Design review of the part built by this model. Coordinates are the model's own, in mm. A direction names the side the tool comes from. Round coordinates to 2 decimals unless told otherwise and drop trailing zeros. Loops run counter-clockwise (first coordinate to the right, second up) from the corner with the lowest first, then second, coordinate; pieces in that order, holes last. Notation, with made-up numbers: M 66,-31.75 L 93,-31.75 A25 ccw 93,-4.75 Z; hole C 16.5,-3 d9. An arc over 180 degrees is marked long. Answer as CSV lines item,"result". Start each with the question number.
Autodesk Fusion 360 part; units mm, degrees
sketch "Sketch1" plane through (0, 0, 0) normal (0, 0, 1) x (1, 0, 0)
  line L0 (5.4842, 0) -> (306.4842, 0)
  line L1 (311.4842, 5) -> (311.4842, 200)
  line L2 (306.4842, 205) -> (5.4842, 205)
  line L3 (0.4842, 200) -> (0.4842, 5)
  line L4 (8.4842, 2.5) -> (303.4842, 2.5)
  line L5 (308.4842, 7.5) -> (308.4842, 197.5)
  line L6 (303.4842, 202.5) -> (8.4842, 202.5)
  line L7 (3.4842, 197.5) -> (3.4842, 7.5)
  arc A0 (8.4842, 202.5) -> (3.4842, 197.5) centre (8.4842, 197.5) ccw
  arc A1 (5.4842, 205) -> (0.4842, 200) centre (5.4842, 200) ccw
  arc A2 (308.4842, 197.5) -> (303.4842, 202.5) centre (303.4842, 197.5) ccw
  arc A3 (311.4842, 200) -> (306.4842, 205) centre (306.4842, 200) ccw
  arc A4 (3.4842, 7.5) -> (8.4842, 2.5) centre (8.4842, 7.5) ccw
  arc A5 (0.4842, 5) -> (5.4842, 0) centre (5.4842, 5) ccw
  arc A6 (303.4842, 2.5) -> (308.4842, 7.5) centre (303.4842, 7.5) ccw
  arc A7 (306.4842, 0) -> (311.4842, 5) centre (306.4842, 5) ccw
  point P0 (0.4842, 0)
  point P1 (311.4842, 0)
  point P2 (3.4842, 2.5)
  point P3 (308.4842, 2.5)
  dimension "d1" = 311
  dimension "d2" = 205
  dimension "d3" = 305
  dimension "d4" = 200
  dimension "d5" = 2.5
  dimension "d6" = 2.5
  dimension "d7" = 3
  dimension "d8" = 3
  dimension "d9" = 5
  dimension "d10" = 5
  dimension "d11" = 5
  dimension "d12" = 5
  dimension "d13" = 5
  dimension "d14" = 5
  dimension "d15" = 5
  dimension "d16" = 5
extrude "Extrude1" add sketch "Sketch1" along normal blind 25
Item 1: Consider section C-C, the plane z = 18.25. Write out the cut boundary in (x, y).
Item 2: Consider section A-A, the plane x = 167.5. Write out the cut boundary in (y, z), then the cut area to 3 significant figures.
Item 3: Consider section B-B, the plane y = 62. Write out the cut boundary in (x, z), then the cut area to 3 significant figures.
Item 4: The part is to be moulded in two halves that separate along X. For faces 1 (the face through (0.484, 104, 12)), 2 (the face through (3.484, 104, 12)), 3 (the face through (311.484, 101, 12)), say which applies: +X half, -X half, draft (parallel to the pull), parting line (faces both ways), or undercut.
Item 5: Tool access review of faces 4 (the face through (154, 0, 12)), 5 (the face through (158, 202.5, 12)): name each direction out of +Z, -Z, +X, -X, +Y, -Y from which nothing blocks a thin tool from reaching the whole face with its end or side.
Item 6: To check wall thickness, follow line 1 (X direction, y = 171, z = 13.5); line 2 (Y direction, x = 168.5, z = 10.25). State the ranges of each line that lie inside material, in increasing order.
Found:
1,outline,"M 0.48,5 A5 ccw 5.48,0 L 306.48,0 A5 ccw 311.48,5 L 311.48,200 A5 ccw 306.48,205 L 5.48,205 A5 ccw 0.48,200 Z; hole M 3.48,7.5 A5 ccw 8.48,2.5 L 303.48,2.5 A5 ccw 308.48,7.5 L 308.48,197.5 A5 ccw 303.48,202.5 L 8.48,202.5 A5 ccw 3.48,197.5 Z"
2,outline,"M 0,0 L 2.5,0 L 2.5,25 L 0,25 Z; M 202.5,0 L 205,0 L 205,25 L 202.5,25 Z"
2,area,"125 mm^2"
3,outline,"M 0.48,0 L 3.48,0 L 3.48,25 L 0.48,25 Z; M 308.48,0 L 311.48,0 L 311.48,25 L 308.48,25 Z"
3,area,"150 mm^2"
4,face 1,"-X half"
4,face 2,"undercut"
4,face 3,"+X half"
5,face 4,"+Z, -Z, +X, -X, -Y"
5,face 5,"+Z, -Z"
6,line 1,"x = 0.48 to 3.48, 308.48 to 311.48"
6,line 2,"y = 0 to 2.5, 202.5 to 205"
